from build123d import *

# Parameters (mm, degrees)
SKETCH1_R           = 19
BOSS_EXTRUDE1_DEPTH = 945
BOSS_EXTRUDE2_START = -110
SKETCH2_R           = 19
BOSS_EXTRUDE2_DEPTH = 110
SKETCH3_R           = 3.175
CUT_EXTRUDE1_DEPTH  = 948.626429889


with BuildPart() as part:
    # Sketch1 → Boss-Extrude1 (new body)
    with BuildSketch(Plane.XY):
        Circle(SKETCH1_R)
    extrude(amount=BOSS_EXTRUDE1_DEPTH)

    # Sketch2 → Boss-Extrude2 (add)
    with BuildSketch(Plane.XY.offset(945).offset(BOSS_EXTRUDE2_START)):
        with BuildLine():
            Line((-60, -9.525), (-25.797759108, -9.525))
            ThreePointArc((-25.797759108, -9.525), (0, -27.5), (25.797759108, -9.525))
            Line((25.797759108, -9.525), (60, -9.525))
            Line((60, -9.525), (60, 9.525))
            Line((60, 9.525), (25.797759108, 9.525))
            ThreePointArc((25.797759108, 9.525), (0, 27.5), (-25.797759108, 9.525))
            Line((-25.797759108, 9.525), (-60, 9.525))
            Line((-60, 9.525), (-60, -9.525))
        make_face()
        Circle(SKETCH2_R, mode=Mode.SUBTRACT)
    extrude(amount=BOSS_EXTRUDE2_DEPTH)

    # Sketch3 → Cut-Extrude1 (cut, through all)
    with BuildSketch(Plane(origin=(0, 9.525, 0), x_dir=(1, 0, 0), z_dir=(0, 1, 0))):
        with Locations(Location((40, -925, 0), (0, 0, 180))):
            Circle(SKETCH3_R)
        with Locations(Location((40, -855, 0), (0, 0, 180))):
            Circle(SKETCH3_R)
        with Locations(Location((-40, -925, 0), (0, 0, 180))):
            Circle(SKETCH3_R)
        with Locations(Location((-40, -855, 0), (0, 0, 180))):
            Circle(SKETCH3_R)
    extrude(amount=-CUT_EXTRUDE1_DEPTH, mode=Mode.SUBTRACT)


solid = part.part
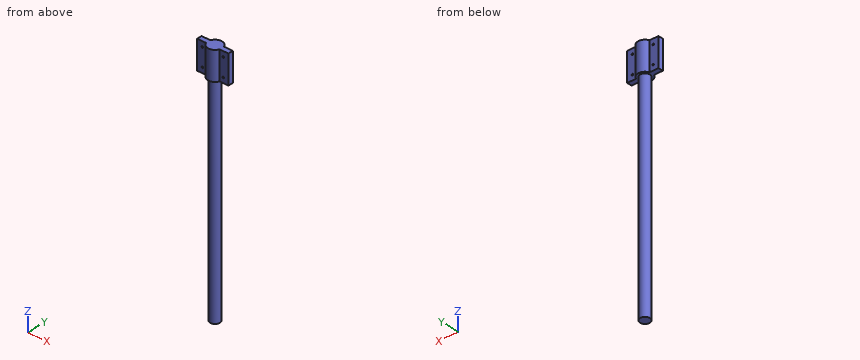
Build history of the part. All positions in model axes, mm. Round coordinates to 2 decimals unless told otherwise and drop trailing zeros. Write each loop counter-clockwise with the first axis right and the second up, starting at its lowest first coordinate (ties: lowest second). Pieces come first, ordered by that corner, then holes. Notation, with made-up numbers: M 56.5,-3.5 L 81.5,-3.5 A18 ccw 81.5,0.5 Z; hole C -14,-31.75 d5. An arc over 180 degrees is marked long. Answer as a JSON object with one key per item and string values. Group by question number.
(1) Cut at B-B (z = 262). Give the cut face in (x, y).
(2) Flat gauge pins, fed straight in: pin 1 (2 mm diameter, centred on x = 1, y = -3, fed in from -Z); pin 2 (7.5 mm diameter, centred on x = 40, z = 855, fed in from -Y) (3 decimals); pin 3 (4 mm diameter, centred on x = -40, z = 855, fed in from -Y); pin 4 (10.5 mm diameter, centred on x = 36, z = 908.5, fed in from +Y) (3 decimals). Where does each tip first touch, or does it go through?
(3) Cut at A-A (x = 0). Give the cut face in (y, z), and give its area (3 significant figures).
(4) Drill centre lines: L1, parallel to Z at x = -40, y = -2.25 (3 decimals); L2, parallel to X at y = 5.75, z = 925 (3 decimals); L3, parallel to Y at x = -2, z = 86.5. Where is each one in solid material? Low to high.
Responses:
{
 "1": {"outline": "C 0,0 d38"},
 "2": {"pin 1": "stops at z = 0", "pin 2": "stops at y = -9.525", "pin 3": "passes through", "pin 4": "stops at y = 9.525"},
 "3": {"outline": "M -27.5,835 L -19,835 L -19,0 L 19,0 L 19,835 L 27.5,835 L 27.5,945 L -27.5,945 Z", "area": "37,800 mm2"},
 "4": {"L1": "z = 835 to 851.825, 858.175 to 921.825, 928.175 to 945", "L2": "x = -60 to -43.175, -36.825 to 36.825, 43.175 to 60", "L3": "y = -18.89 to 18.89"}
}
